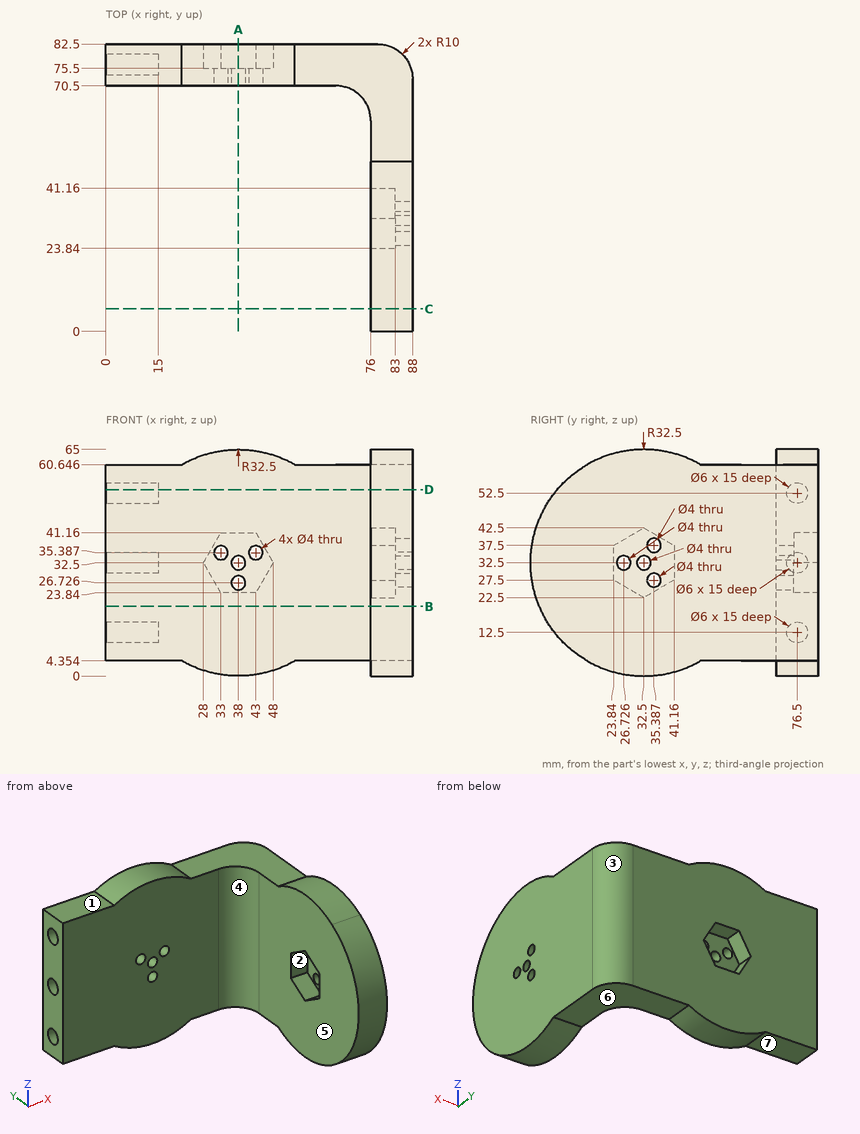
Could you check a few things on this drawing? It's one solid part, dimensions in mm from its lowest x, y, z. A direction names the side the tool comes from. Round coordinates to 2 decimals unless told otherwise and drop trailing zeros. Loops run counter-clockwise (first coordinate to the right, second up) from the corner with the lowest first, then second, coordinate; pieces in that order, holes last. Notation, with made-up numbers: (70, 47) -> (96, 47) arc R15 cw to (96, 54) -> close; hole circle Ø5 at (12, -10.5). An arc over 180 degrees is marked (long way). Answer as CSV lines item,"result".
1. If we section it at C-C on y = 6.5: Please give me the cut outline in (x, z).
Final values:
outline,"(76, 13) -> (88, 13) -> (88, 52) -> (76, 52) -> close"
2. If we section it at B-B on z = 20: Please give me the cut outline in (x, y), plus the area to 3 significant figures.
Final values:
outline,"(0, 70.5) -> (66, 70.5) arc R10 cw to (76, 60.5) -> (76, 2.5) -> (88, 2.5) -> (88, 72.5) arc R10 ccw to (78, 82.5) -> (0, 82.5) -> close"
area,"1,870 mm^2"
3. If we section it at D-D on z = 53.5: Please give me the cut outline in (x, y) (1 decimal).
Final values:
outline,"(0, 70.5) -> (66, 70.5) arc R10 cw to (76, 60.5) -> (76, 7.7) -> (88, 7.7) -> (88, 72.5) arc R10 ccw to (78, 82.5) -> (0, 82.5) -> (0, 79.3) -> (15, 79.3) -> (15, 73.7) -> (0, 73.7) -> close"
4. Which directions (+Z, -Z, +X, -X, +Y, -Y) give clear straight access to the entire face, cutting with the end or side of a thin tool? Please do the marked faces 5, 6 and 7.
Final values:
face 5,"+Z, -Z, -X, -Y"
face 6,"-Z, +X, +Y"
face 7,"-Z, -X, +Y, -Y"
5. Thinking about a two-plate mould opening in Y: for the marked faces 1, 2, 3 and 4, which applies, released by +Y, released by -Y, zero draft, split by the parting line, or undercut?
Final values:
face 1,"zero draft"
face 2,"undercut"
face 3,"released by +Y"
face 4,"released by -Y"
6. If I drill on L1, parallel to Y at x = 10, z = 52.5; L2, parallel to X at y = 25, z = 22; L3, parallel to Y at x = 25, z = 41, over which ranges is the centre line in solid material (lowest first)?
Final values:
L1,"y = 70.5 to 73.5, 79.5 to 82.5"
L2,"x = 76 to 88"
L3,"y = 70.5 to 82.5"
7. If we section it at A-A on x = 38: Please give me the cut outline in (y, z), plus the area to 3 significant figures.
Final values:
outline,"(70.5, 0) -> (82.5, 0) -> (82.5, 23.84) -> (75.5, 23.84) -> (75.5, 24.73) -> (70.5, 24.73) -> close; (70.5, 28.73) -> (75.5, 28.73) -> (75.5, 30.5) -> (70.5, 30.5) -> close; (70.5, 34.5) -> (75.5, 34.5) -> (75.5, 41.16) -> (82.5, 41.16) -> (82.5, 65) -> (70.5, 65) -> close"
area,"619 mm^2"
8. For pin 1 (14 mm diameter, centred on x = 38.5, z = 32, fed in from +Y); pin 2 (13 mm diameter, centred on x = 8, y = 74.5, fed in from -Z); pin 3 (1.8 mm diameter, centred on y = 76, z = 52.5, fed in from -X), each with a flat end and sliding along its axis, tell me the tip position at first contact or that it passes through.
Final values:
pin 1,"stops at y = 75.5"
pin 2,"stops at z = 4.35"
pin 3,"stops at x = 15"
